```python
from build123d import *

# Parameters (mm, degrees)
F0_R     = 1
F0_W     = 20
F0_H     = 15
F0_H_2   = 20
F0_R_2   = 1.9
F1_DEPTH = 10
F2_R     = 1.75
F3_DEPTH = 60.001
F4_W     = 2
F4_H     = 20.12
F5_DEPTH = 70.001
F6_R     = 1.45
F7_DEPTH = 8.001
F8_DEPTH = 35
F9_SIZE  = 5
F10_SIZE = 2


with BuildPart() as f1:
    # F0 (on Front) → F1 (new body)
    with BuildSketch(Plane.XZ):
        Polygon((35, 40), (-35, 40), (-35, 0), (-10, 0), (10, 0), (35, 0), align=None)
        with Locations((-31, 3.5)):
            Circle(F0_R, mode=Mode.SUBTRACT)
        with Locations((-26.5, 6.5)):
            Circle(F0_R, mode=Mode.SUBTRACT)
        with Locations((-13.5, 6.5)):
            Circle(F0_R, mode=Mode.SUBTRACT)
        with Locations((12, 7)):
            Circle(F0_R, mode=Mode.SUBTRACT)
        with Locations((31, 3.5)):
            Circle(F0_R, mode=Mode.SUBTRACT)
        with Locations((-28.25, 37)):
            Circle(F0_R, mode=Mode.SUBTRACT)
        with Locations((-11.75, 37)):
            Circle(F0_R, mode=Mode.SUBTRACT)
        with Locations((0, 12.5)):
            Rectangle(F0_W, F0_H, mode=Mode.SUBTRACT)
        with Locations((12, 30)):
            Circle(F0_R, mode=Mode.SUBTRACT)
        with Locations((10, 36.5)):
            Circle(F0_R, mode=Mode.SUBTRACT)
        with Locations((0, -10)):
            Rectangle(F0_W, F0_H_2)
        with Locations((0, -13.5)):
            Circle(F0_R_2, mode=Mode.SUBTRACT)
    extrude(amount=F1_DEPTH)

    # F2 (on face) → F3 (cut, through all)
    with BuildSketch(Plane.XY.offset(40)):
        with Locations((-20, -5)):
            Circle(F2_R)
        with Locations((20, -5)):
            Circle(F2_R)
    extrude(amount=-F3_DEPTH, mode=Mode.SUBTRACT)

    # F4 (on face) → F5 (cut, through all)
    with BuildSketch(Plane(origin=(-35, 0, 0), x_dir=(0, -1, 0), z_dir=(-1, 0, 0))):
        with Locations((9, 25)):
            Rectangle(F4_W, F4_H)
    extrude(amount=-F5_DEPTH, mode=Mode.SUBTRACT)

    # F6 (on face) → F7 (cut, through all)
    with BuildSketch(Plane.XZ.offset(8)):
        with Locations((0, 25)):
            Circle(F6_R)
    extrude(amount=-F7_DEPTH, mode=Mode.SUBTRACT)

    # F2 (on face) → F8 (cut)
    with BuildSketch(Plane.XY.offset(40)):
        with Locations((-20, -5)):
            Circle(F2_R)
        with Locations((20, -5)):
            Circle(F2_R)
        with BuildLine():
            Line((-24, -5), (-24, -10))
            Line((-24, -10), (-16, -10))
            Line((-16, -10), (-16, -5))
            ThreePointArc((-16, -5), (-20, -1), (-24, -5))
        make_face()
        with Locations((-20, -5)):
            Circle(F2_R, mode=Mode.SUBTRACT)
        with BuildLine():
            Line((16, -5), (16, -10))
            Line((16, -10), (24, -10))
            Line((24, -10), (24, -5))
            ThreePointArc((24, -5), (20, -1), (16, -5))
        make_face()
        with Locations((20, -5)):
            Circle(F2_R, mode=Mode.SUBTRACT)
    extrude(amount=-F8_DEPTH, mode=Mode.SUBTRACT)

    # F9
    f9_edges = [f1.edges().sort_by_distance(p)[0] for p in [
        (10, -5, -20),
        (-10, -5, -20),
    ]]
    chamfer(f9_edges, length=F9_SIZE)

    # F10
    f10_edges = [f1.edges().sort_by_distance(p)[0] for p in [
        (-35, -5, 40),
        (35, -5, 40),
    ]]
    chamfer(f10_edges, length=F10_SIZE)


solid = f1.part
```
For this review, take the finished solid that the model builds, in its own axes (mm). A direction names the side the tool comes from. Coordinates: 2 decimals unless noted, no trailing zeros. Order: outer loops, then holes, each group sorted by start corner. A loop starts at its lowest first (then second) coordinate and runs counter-clockwise, first axis right, second up. Notation, with made-up numbers: (-17.75, 86.5) - (35.25, 86.5) arc R35 cw to (35.25, 122.5) - close; hole circle Ø6 at (12, 4). An arc over 180 degrees is marked (long way). Answer as a JSON object with one key per item and string values. Group by question number.
1. For faces 1 (the flat face through (10, -5, -8)), 2 (the flat face through (-34, -5, 39)), 3 (the flat face through (10, -5, 12)), 4 (the flat face through (-30, -9, 35.06)), list the 3-axis set-ups (+Z, -Z, +X, -X, +Y, -Y) from which the entire face can be reached by the end or side of a thin tool; tool diameter is ignored.
2. We need section D-D on x = -13.5. State the section outline as (y, z) points.
3. For probe 1 along X at (y, z) = (-5, 34); probe 2 along Z at (x, y) = (0, -4.75); probe 3 along X at (y, z) = (-5, 19.5), list the stretches that pass through material, from the lowest coordinate up.
4. We need section A-A on z = -13.5. State the section outline as (x, y) points, then the cut area to 3 significant figures.
5. The part is to be moulded in two halves that separate along Z. For faces 5 (the flat face through (-20, -7, 5)), 6 (the cylindrical face through (-11.88, -4.93, 37.99)), 7 (the flat face through (22, -5, 0)), say which applies: pulls with the +Z half, pulls with the -Z half, needs draft (parallel to the pull), parting line crosses it, or undercut.
6. We need section C-C on x = 0. State the section outline as (y, z) points.
7. We need section B-B on x = 12. State the section outline as (y, z) points, then the cut area to 3 significant figures.
8. Clearance check with flat-ended pins moving along their axes: P1, Ø1.6, axis at x = 12, z = 7, coming from the +Y side; P2, Ø10, axis at x = -5, z = 30, coming from the -Y side; P3, Ø0.6, axis at x = 27.5, y = -9, coming from the -Z side; P4, Ø1.5, axis at x = -19, y = -7, coming from the +Z side. State where each tip first meets the part, or that it passes through.
Final values:
{
 "1": {"face 1": "-Z, +X, +Y, -Y", "face 2": "+Z, -X, +Y, -Y", "face 3": "+Y, -Y", "face 4": "+X, -X, -Y"},
 "2": {"outline": "(-10, 0) - (0, 0) - (0, 5.5) - (-10, 5.5) - close; (-10, 7.5) - (0, 7.5) - (0, 40) - (-10, 40) - (-10, 35.06) - (-8, 35.06) - (-8, 14.94) - (-10, 14.94) - close"},
 "3": {"probe 1": "-35 to -24, -16 to 16, 24 to 35", "probe 2": "-20 to -15.4, -11.6 to 5, 20 to 23.55, 26.45 to 40", "probe 3": "-35 to -24, -16 to -10, 10 to 16, 24 to 35"},
 "4": {"outline": "(-10, -10) - (-1.9, -10) - (-1.9, 0) - (-10, 0) - close; (1.9, -10) - (10, -10) - (10, 0) - (1.9, 0) - close", "area": "162 mm²"},
 "5": {"face 5": "pulls with the +Z half", "face 6": "undercut", "face 7": "pulls with the -Z half"},
 "6": {"outline": "(-10, -20) - (0, -20) - (0, -15.4) - (-10, -15.4) - close; (-10, -11.6) - (0, -11.6) - (0, 5) - (-10, 5) - close; (-10, 35.06) - (-8, 35.06) - (-8, 26.45) - (0, 26.45) - (0, 40) - (-10, 40) - close; (-8, 20) - (0, 20) - (0, 23.55) - (-8, 23.55) - close"},
 "7": {"outline": "(-10, 0) - (0, 0) - (0, 6) - (-10, 6) - close; (-10, 8) - (0, 8) - (0, 29) - (-8, 29) - (-8, 14.94) - (-10, 14.94) - close; (-10, 35.06) - (-8, 35.06) - (-8, 31) - (0, 31) - (0, 40) - (-10, 40) - close", "area": "324 mm²"},
 "8": {"P1": "through", "P2": "y = -8", "P3": "z = 0", "P4": "z = 5"}
}
